```python
from build123d import *

# Parameters (mm, degrees)
EXTRUDE1_DEPTH                               = 3
CSK_FOR_M4_COUNTERSUNK_FLAT_HEAD_SCR_2_COUNT = 2
CSK_FOR_M4_COUNTERSUNK_FLAT_HEAD_SCR_2_PITCH = 81
CSK_FOR_M4_COUNTERSUNK_FLAT_HEAD_SCR_3_COUNT = 2
CSK_FOR_M4_COUNTERSUNK_FLAT_HEAD_SCR_3_PITCH = 58.523499554
CSK_FOR_M4_COUNTERSUNK_FLAT_HEAD_SCR_4_COUNT = 2
CSK_FOR_M4_COUNTERSUNK_FLAT_HEAD_SCR_4_PITCH = 32
CSK_FOR_M4_COUNTERSUNK_FLAT_HEAD_SCR_5_COUNT = 2
CSK_FOR_M4_COUNTERSUNK_FLAT_HEAD_SCR_5_PITCH = 113.159179919
CSK_FOR_M4_COUNTERSUNK_FLAT_HEAD_SCR_6_COUNT = 2
CSK_FOR_M4_COUNTERSUNK_FLAT_HEAD_SCR_6_PITCH = 130.249760077
CSK_FOR_M4_COUNTERSUNK_FLAT_HEAD_SCR_7_COUNT = 2
CSK_FOR_M4_COUNTERSUNK_FLAT_HEAD_SCR_7_PITCH = 189.179808648
CSK_FOR_M4_COUNTERSUNK_FLAT_HEAD_SCR_8_COUNT = 2
CSK_FOR_M4_COUNTERSUNK_FLAT_HEAD_SCR_8_PITCH = 218.387270691
CSK_FOR_M4_COUNTERSUNK_FLAT_HEAD_SCR_9_COUNT = 2
CSK_FOR_M4_COUNTERSUNK_FLAT_HEAD_SCR_9_PITCH = 207.858124691
FILLET1_R                                    = 3


with BuildPart() as part:
    # Sketch1 → Extrude1 (new body)
    with BuildSketch(Plane(origin=(0, 0, 0), x_dir=(1, 0, 0), z_dir=(0, 1, 0))):
        Polygon((0, 0), (220, 0), (220, 47.5), (55, 47.5), (55, 100), (0, 100), align=None)
    extrude(amount=EXTRUDE1_DEPTH)

    # Sketch3 → CSK for M4 Countersunk Flat Head Screw1 (revolve, cut)
    with BuildSketch(Plane(origin=(11.5, 3, -90), x_dir=(0, 0, 1), z_dir=(1, 0, 0))):
        Polygon((0, 0), (0, 3), (2.25, 3), (2.25, 2.45), (4.7, 0), align=None)
    csk_for_m4_countersunk_flat_head_screw1 = revolve(axis=Axis((11.5, 9.35, -90), (0, -1, 0)), mode=Mode.SUBTRACT)

    # CSK for M4 Countersunk Flat Head Scr 2: CSK for M4 Countersunk Flat Head Screw1 ×2
    with Locations(*[(0, 0, i * CSK_FOR_M4_COUNTERSUNK_FLAT_HEAD_SCR_2_PITCH) for i in range(1, CSK_FOR_M4_COUNTERSUNK_FLAT_HEAD_SCR_2_COUNT)]):
        add(csk_for_m4_countersunk_flat_head_screw1, mode=Mode.SUBTRACT)

    # CSK for M4 Countersunk Flat Head Scr 3: CSK for M4 Countersunk Flat Head Screw1 ×2
    with Locations(*[Vector(0.546788901, 0, 0.837270505) * (i * CSK_FOR_M4_COUNTERSUNK_FLAT_HEAD_SCR_3_PITCH) for i in range(1, CSK_FOR_M4_COUNTERSUNK_FLAT_HEAD_SCR_3_COUNT)]):
        add(csk_for_m4_countersunk_flat_head_screw1, mode=Mode.SUBTRACT)

    # CSK for M4 Countersunk Flat Head Scr 4: CSK for M4 Countersunk Flat Head Screw1 ×2
    with Locations(*[(i * CSK_FOR_M4_COUNTERSUNK_FLAT_HEAD_SCR_4_PITCH, 0, 0) for i in range(1, CSK_FOR_M4_COUNTERSUNK_FLAT_HEAD_SCR_4_COUNT)]):
        add(csk_for_m4_countersunk_flat_head_screw1, mode=Mode.SUBTRACT)

    # CSK for M4 Countersunk Flat Head Scr 5: CSK for M4 Countersunk Flat Head Screw1 ×2
    with Locations(*[Vector(0.901385111, 0, 0.433018338) * (i * CSK_FOR_M4_COUNTERSUNK_FLAT_HEAD_SCR_5_PITCH) for i in range(1, CSK_FOR_M4_COUNTERSUNK_FLAT_HEAD_SCR_5_COUNT)]):
        add(csk_for_m4_countersunk_flat_head_screw1, mode=Mode.SUBTRACT)

    # CSK for M4 Countersunk Flat Head Scr 6: CSK for M4 Countersunk Flat Head Screw1 ×2
    with Locations(*[Vector(0.783110847, 0, 0.621882144) * (i * CSK_FOR_M4_COUNTERSUNK_FLAT_HEAD_SCR_6_PITCH) for i in range(1, CSK_FOR_M4_COUNTERSUNK_FLAT_HEAD_SCR_6_COUNT)]):
        add(csk_for_m4_countersunk_flat_head_screw1, mode=Mode.SUBTRACT)

    # CSK for M4 Countersunk Flat Head Scr 7: CSK for M4 Countersunk Flat Head Screw1 ×2
    with Locations(*[Vector(0.898615985, 0, 0.43873604) * (i * CSK_FOR_M4_COUNTERSUNK_FLAT_HEAD_SCR_7_PITCH) for i in range(1, CSK_FOR_M4_COUNTERSUNK_FLAT_HEAD_SCR_7_COUNT)]):
        add(csk_for_m4_countersunk_flat_head_screw1, mode=Mode.SUBTRACT)

    # CSK for M4 Countersunk Flat Head Scr 8: CSK for M4 Countersunk Flat Head Screw1 ×2
    with Locations(*[Vector(0.924962336, 0, 0.380058782) * (i * CSK_FOR_M4_COUNTERSUNK_FLAT_HEAD_SCR_8_PITCH) for i in range(1, CSK_FOR_M4_COUNTERSUNK_FLAT_HEAD_SCR_8_COUNT)]):
        add(csk_for_m4_countersunk_flat_head_screw1, mode=Mode.SUBTRACT)

    # CSK for M4 Countersunk Flat Head Scr 9: CSK for M4 Countersunk Flat Head Screw1 ×2
    with Locations(*[Vector(0.971816715, 0, 0.235737718) * (i * CSK_FOR_M4_COUNTERSUNK_FLAT_HEAD_SCR_9_PITCH) for i in range(1, CSK_FOR_M4_COUNTERSUNK_FLAT_HEAD_SCR_9_COUNT)]):
        add(csk_for_m4_countersunk_flat_head_screw1, mode=Mode.SUBTRACT)

    # Fillet1
    fillet1_edges = [part.edges().sort_by_distance(p)[0] for p in [
        (0, 1.5, -100),
        (55, 1.5, -100),
        (55, 1.5, -47.5),
        (220, 1.5, -47.5),
        (0, 1.5, 0),
    ]]
    fillet(fillet1_edges, radius=FILLET1_R)


solid = part.part
```
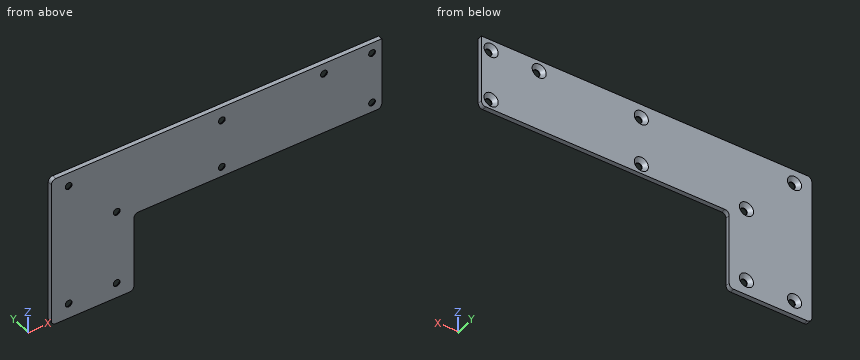
Check sheet for the modelled part. Datum: model origin and axes. Units: mm. Coordinates: 2 decimals unless noted, no trailing zeros. Order: outer loops, then holes, each group sorted by start corner. A loop starts at its lowest first (then second) coordinate and runs counter-clockwise, first axis right, second up. Notation, with made-up numbers: M 66,-24 L 120,-24 A23 ccw 120,0 Z; hole C 86,42.5 d7. An arc over 180 degrees is marked long. Write each question's results on one line, items separated by ' | '. Start each with the question number.
1. Material ranges on probe 1 along X at (y, z) = (0.25, -41); probe 2 along Z at (x, y) = (11.5, 0.3); probe 3 along Z at (x, y) = (113.5, 0.45), recorded low to high.
2. Cross-section at B-B on z = -41. Record the cut outline in (x, y).
3. Go/stop test with flat-tipped pins: P1, Ø4, axis at x = 181.5, z = -7, coming from the +Y side; P2, Ø5, axis at x = 11.5, z = -90, coming from the +Y side; P3, Ø7, axis at x = 11.5, z = -9, coming from the +Y side; P4, Ø6, axis at x = 213.5, z = -41, coming from the +Y side. Record where each tip stops, or that it passes through.
4. Cross-section at A-A on x = 113.5. Record the cut outline in (y, z).
5. Cross-section at D-D on x = 181.5. Record the cut outline in (y, z).
6. Cross-section at C-C on y = 1.9. State how many separate pieces and enclosed holes the cut face has, and give its area (3 significant figures).
Checks:
1) probe 1: x = 0 to 41.25, 45.75 to 111.25, 115.75 to 211.25, 215.75 to 220 | probe 2: z = -100 to -92.25, -87.75 to -11.25, -6.75 to 0 | probe 3: z = -47.5 to -43.25, -38.75 to -11.25, -6.75 to 0
2) outline: M 0,0 L 41.25,0 L 41.25,0.55 L 38.8,3 L 0,3 Z; M 45.75,0 L 111.25,0 L 111.25,0.55 L 108.8,3 L 48.2,3 L 45.75,0.55 Z; M 115.75,0 L 211.25,0 L 211.25,0.55 L 208.8,3 L 118.2,3 L 115.75,0.55 Z; M 215.75,0 L 220,0 L 220,3 L 218.2,3 L 215.75,0.55 Z
3) P1: passes through | P2: stops at y = 0.8 | P3: stops at y = 1.8 | P4: stops at y = 1.3
4) outline: M 0,-47.5 L 3,-47.5 L 3,-45.7 L 0.55,-43.25 L 0,-43.25 Z; M 0,-38.75 L 0.55,-38.75 L 3,-36.3 L 3,-13.7 L 0.55,-11.25 L 0,-11.25 Z; M 0,-6.75 L 0.55,-6.75 L 3,-4.3 L 3,0 L 0,0 Z
5) outline: M 0,-47.5 L 3,-47.5 L 3,-11.7 L 0.55,-9.25 L 0,-9.25 Z; M 0,-4.75 L 0.55,-4.75 L 3,-2.3 L 3,0 L 0,0 Z
6) separate pieces: 1 | enclosed holes: 9 | area: 13,000 mm²
